from build123d import *

# Parameters (mm, degrees)
BOSS_EXTRUDE1_DEPTH      = 48
CUT_EXTRUDE4_DEPTH       = 2
CUT_EXTRUDE6_DEPTH       = 9
CUT_EXTRUDE6_DEPTH_BACK  = 1
SKETCH8_RX               = 1.5
SKETCH8_RY               = 0.8
CUT_EXTRUDE7_DEPTH       = 11
CUT_EXTRUDE7_DEPTH_BACK  = 1
SKETCH13_RX              = 1.5
SKETCH13_RY              = 0.8
CUT_EXTRUDE8_DEPTH       = 13
CUT_EXTRUDE8_DEPTH_BACK  = 1
SKETCH14_RX              = 1.5
SKETCH14_RY              = 0.8
CUT_EXTRUDE9_DEPTH       = 15
CUT_EXTRUDE9_DEPTH_BACK  = 1
SKETCH15_RX              = 1.5
SKETCH15_RY              = 0.8
CUT_EXTRUDE10_DEPTH      = 17
CUT_EXTRUDE10_DEPTH_BACK = 1
SKETCH16_RX              = 1.5
SKETCH16_RY              = 0.8
CUT_EXTRUDE11_DEPTH      = 19
CUT_EXTRUDE11_DEPTH_BACK = 1
SKETCH17_RX              = 1.5
SKETCH17_RY              = 0.8
CUT_EXTRUDE12_DEPTH      = 21
CUT_EXTRUDE12_DEPTH_BACK = 1
SKETCH18_RX              = 1.5
SKETCH18_RY              = 0.8
CUT_EXTRUDE13_DEPTH      = 23
CUT_EXTRUDE13_DEPTH_BACK = 1
SKETCH19_RX              = 1.5
SKETCH19_RY              = 0.8
SKETCH21_W               = 58.141640115
SKETCH21_H               = 26.059597095
CUT_EXTRUDE14_DEPTH      = 22
BODY_MOVE_COPY1_ANGLE    = 180


with BuildPart() as part:
    # Sketch2 → Boss-Extrude1 (new body)
    with BuildSketch(Plane.XY):
        Polygon((-7.23, -20.3), (-7.23, -34), (-9.23, -34), (-9.23, -2), (-7.23, -2), align=None)
    extrude(amount=BOSS_EXTRUDE1_DEPTH)

    # Sketch7 → Cut-Extrude4 (cut)
    with BuildSketch(Plane(origin=(-7.23, 0, 0), x_dir=(0, 0, -1), z_dir=(1, 0, 0))):
        Polygon((-48, -16.3), (-48, -24.3), (-42, -24.3), (-42, -25.3), (-36, -25.3), (-36, -26.3), (-30, -26.3), (-30, -27.3), (-24, -27.3), (-24, -28.3), (-18, -28.3), (-18, -29.3), (-12, -29.3), (-12, -30.3), (-6, -30.3), (-6, -31.3), (0, -31.3), (0, -9.3), (-6, -9.3), (-6, -10.3), (-12, -10.3), (-12, -11.3), (-18, -11.3), (-18, -12.3), (-24, -12.3), (-24, -13.3), (-30, -13.3), (-30, -14.3), (-36, -14.3), (-36, -15.3), (-42, -15.3), (-42, -16.3), align=None)
    extrude(amount=-CUT_EXTRUDE4_DEPTH, mode=Mode.SUBTRACT)


with BuildPart() as cut_extrude4_piece_1:
    # of the separate pieces the step leaves, piece 1, a body of its own (cut_extrude4_pieces)
    add(part.part.solids().sort_by_distance((-7.23, -9.3, 0))[0])


with BuildPart() as cut_extrude4_piece_2:
    # of the separate pieces the step leaves, piece 2, a body of its own (cut_extrude4_pieces)
    add(part.part.solids().sort_by_distance((-7.23, -34, 0))[0])


with BuildPart() as cut_extrude6_tool:
    # Sketch8 → Cut-Extrude6 (new, two sides: drawn at the far end of the back side and taken through both)
    with BuildSketch(Plane(origin=(0, -24.3, 0), x_dir=(1, 0, 0), z_dir=(0, 1, 0)).offset(-CUT_EXTRUDE6_DEPTH_BACK)):
        with Locations(Location((-8.23, -45), (0, 0, 90))):
            Ellipse(SKETCH8_RX, SKETCH8_RY)
    extrude(amount=CUT_EXTRUDE6_DEPTH + CUT_EXTRUDE6_DEPTH_BACK)


with BuildPart() as cut_extrude4_piece_1_1:
    add(cut_extrude4_piece_1.part)

    # Cut-Extrude6: cut by cut_extrude6_tool
    add(cut_extrude6_tool.part, mode=Mode.SUBTRACT)


with BuildPart() as cut_extrude4_piece_2_1:
    add(cut_extrude4_piece_2.part)

    # Cut-Extrude6: cut by cut_extrude6_tool
    add(cut_extrude6_tool.part, mode=Mode.SUBTRACT)


with BuildPart() as cut_extrude7_tool:
    # Sketch13 → Cut-Extrude7 (new, two sides: drawn at the far end of the back side and taken through both)
    with BuildSketch(Plane(origin=(0, -25.3, 0), x_dir=(1, 0, 0), z_dir=(0, 1, 0)).offset(-CUT_EXTRUDE7_DEPTH_BACK)):
        with Locations(Location((-8.23, -39), (0, 0, 90))):
            Ellipse(SKETCH13_RX, SKETCH13_RY)
    extrude(amount=CUT_EXTRUDE7_DEPTH + CUT_EXTRUDE7_DEPTH_BACK)


with BuildPart() as cut_extrude4_piece_1_2:
    add(cut_extrude4_piece_1_1.part)

    # Cut-Extrude7: cut by cut_extrude7_tool
    add(cut_extrude7_tool.part, mode=Mode.SUBTRACT)


with BuildPart() as cut_extrude4_piece_2_2:
    add(cut_extrude4_piece_2_1.part)

    # Cut-Extrude7: cut by cut_extrude7_tool
    add(cut_extrude7_tool.part, mode=Mode.SUBTRACT)


with BuildPart() as cut_extrude8_tool:
    # Sketch14 → Cut-Extrude8 (new, two sides: drawn at the far end of the back side and taken through both)
    with BuildSketch(Plane(origin=(0, -26.3, 0), x_dir=(1, 0, 0), z_dir=(0, 1, 0)).offset(-CUT_EXTRUDE8_DEPTH_BACK)):
        with Locations(Location((-8.23, -33), (0, 0, 90))):
            Ellipse(SKETCH14_RX, SKETCH14_RY)
    extrude(amount=CUT_EXTRUDE8_DEPTH + CUT_EXTRUDE8_DEPTH_BACK)


with BuildPart() as cut_extrude4_piece_1_3:
    add(cut_extrude4_piece_1_2.part)

    # Cut-Extrude8: cut by cut_extrude8_tool
    add(cut_extrude8_tool.part, mode=Mode.SUBTRACT)


with BuildPart() as cut_extrude4_piece_2_3:
    add(cut_extrude4_piece_2_2.part)

    # Cut-Extrude8: cut by cut_extrude8_tool
    add(cut_extrude8_tool.part, mode=Mode.SUBTRACT)


with BuildPart() as cut_extrude9_tool:
    # Sketch15 → Cut-Extrude9 (new, two sides: drawn at the far end of the back side and taken through both)
    with BuildSketch(Plane(origin=(0, -27.3, 0), x_dir=(1, 0, 0), z_dir=(0, 1, 0)).offset(-CUT_EXTRUDE9_DEPTH_BACK)):
        with Locations(Location((-8.23, -27), (0, 0, 90))):
            Ellipse(SKETCH15_RX, SKETCH15_RY)
    extrude(amount=CUT_EXTRUDE9_DEPTH + CUT_EXTRUDE9_DEPTH_BACK)


with BuildPart() as cut_extrude4_piece_1_4:
    add(cut_extrude4_piece_1_3.part)

    # Cut-Extrude9: cut by cut_extrude9_tool
    add(cut_extrude9_tool.part, mode=Mode.SUBTRACT)


with BuildPart() as cut_extrude4_piece_2_4:
    add(cut_extrude4_piece_2_3.part)

    # Cut-Extrude9: cut by cut_extrude9_tool
    add(cut_extrude9_tool.part, mode=Mode.SUBTRACT)


with BuildPart() as cut_extrude10_tool:
    # Sketch16 → Cut-Extrude10 (new, two sides: drawn at the far end of the back side and taken through both)
    with BuildSketch(Plane(origin=(0, -28.3, 0), x_dir=(1, 0, 0), z_dir=(0, 1, 0)).offset(-CUT_EXTRUDE10_DEPTH_BACK)):
        with Locations(Location((-8.23, -21), (0, 0, 90))):
            Ellipse(SKETCH16_RX, SKETCH16_RY)
    extrude(amount=CUT_EXTRUDE10_DEPTH + CUT_EXTRUDE10_DEPTH_BACK)


with BuildPart() as cut_extrude4_piece_1_5:
    add(cut_extrude4_piece_1_4.part)

    # Cut-Extrude10: cut by cut_extrude10_tool
    add(cut_extrude10_tool.part, mode=Mode.SUBTRACT)


with BuildPart() as cut_extrude4_piece_2_5:
    add(cut_extrude4_piece_2_4.part)

    # Cut-Extrude10: cut by cut_extrude10_tool
    add(cut_extrude10_tool.part, mode=Mode.SUBTRACT)


with BuildPart() as cut_extrude11_tool:
    # Sketch17 → Cut-Extrude11 (new, two sides: drawn at the far end of the back side and taken through both)
    with BuildSketch(Plane(origin=(0, -29.3, 0), x_dir=(1, 0, 0), z_dir=(0, 1, 0)).offset(-CUT_EXTRUDE11_DEPTH_BACK)):
        with Locations(Location((-8.23, -15), (0, 0, 90))):
            Ellipse(SKETCH17_RX, SKETCH17_RY)
    extrude(amount=CUT_EXTRUDE11_DEPTH + CUT_EXTRUDE11_DEPTH_BACK)


with BuildPart() as cut_extrude4_piece_1_6:
    add(cut_extrude4_piece_1_5.part)

    # Cut-Extrude11: cut by cut_extrude11_tool
    add(cut_extrude11_tool.part, mode=Mode.SUBTRACT)


with BuildPart() as cut_extrude4_piece_2_6:
    add(cut_extrude4_piece_2_5.part)

    # Cut-Extrude11: cut by cut_extrude11_tool
    add(cut_extrude11_tool.part, mode=Mode.SUBTRACT)


with BuildPart() as cut_extrude12_tool:
    # Sketch18 → Cut-Extrude12 (new, two sides: drawn at the far end of the back side and taken through both)
    with BuildSketch(Plane(origin=(0, -30.3, 0), x_dir=(1, 0, 0), z_dir=(0, 1, 0)).offset(-CUT_EXTRUDE12_DEPTH_BACK)):
        with Locations(Location((-8.23, -9), (0, 0, 90))):
            Ellipse(SKETCH18_RX, SKETCH18_RY)
    extrude(amount=CUT_EXTRUDE12_DEPTH + CUT_EXTRUDE12_DEPTH_BACK)


with BuildPart() as cut_extrude4_piece_1_7:
    add(cut_extrude4_piece_1_6.part)

    # Cut-Extrude12: cut by cut_extrude12_tool
    add(cut_extrude12_tool.part, mode=Mode.SUBTRACT)


with BuildPart() as cut_extrude4_piece_2_7:
    add(cut_extrude4_piece_2_6.part)

    # Cut-Extrude12: cut by cut_extrude12_tool
    add(cut_extrude12_tool.part, mode=Mode.SUBTRACT)


with BuildPart() as cut_extrude13_tool:
    # Sketch19 → Cut-Extrude13 (new, two sides: drawn at the far end of the back side and taken through both)
    with BuildSketch(Plane(origin=(0, -31.3, 0), x_dir=(1, 0, 0), z_dir=(0, 1, 0)).offset(-CUT_EXTRUDE13_DEPTH_BACK)):
        with Locations(Location((-8.23, -3), (0, 0, 90))):
            Ellipse(SKETCH19_RX, SKETCH19_RY)
    extrude(amount=CUT_EXTRUDE13_DEPTH + CUT_EXTRUDE13_DEPTH_BACK)


with BuildPart() as cut_extrude4_piece_1_8:
    add(cut_extrude4_piece_1_7.part)

    # Cut-Extrude13: cut by cut_extrude13_tool
    add(cut_extrude13_tool.part, mode=Mode.SUBTRACT)


with BuildPart() as cut_extrude4_piece_2_8:
    add(cut_extrude4_piece_2_7.part)

    # Cut-Extrude13: cut by cut_extrude13_tool
    add(cut_extrude13_tool.part, mode=Mode.SUBTRACT)

    # Sketch21 → Cut-Extrude14 (cut)
    with BuildSketch(Plane(origin=(0, 0, 0), x_dir=(0, 0, -1), z_dir=(1, 0, 0))):
        with Locations((-20.055207527, -35.194061722)):
            Rectangle(SKETCH21_W, SKETCH21_H)
    extrude(amount=-CUT_EXTRUDE14_DEPTH, mode=Mode.SUBTRACT)


with BuildPart() as cut_extrude4_piece_1_9:
    # Body-Move/Copy1: moved
    add(cut_extrude4_piece_1_8.part.rotate(Axis((-8.23, -9.15, 0), (0, 0, 1)), BODY_MOVE_COPY1_ANGLE))


solid = cut_extrude4_piece_1_9.part
Work out the finished part from the listing and answer in its coordinate system (mm). A direction names the side the tool comes from. Give positions to 0.01 mm unless a question says otherwise; leave off trailing zeros. Write each loop counter-clockwise with the first axis right and the second up, starting at its lowest first coordinate (ties: lowest second). Pieces come first, ordered by that corner, then holes. Notation, with made-up numbers: (40, -34.5) - (79, -34.5) arc R24 cw to (79, -8.5) - close; hole circle Ø5 at (-11.75, -37.5). An arc over 180 degrees is marked (long way). One line per item, written item: value. Start each with the question number.
1. For a pull along X with two mould halves and no side action, classify faces 1 (the flat face through (-9, -6, 20)), 2 (the flat face through (-8, -4, 39)), 3 (the flat face through (-7.23, -11, 24)) as +X half, -X half, draft (parallel to the pull), parting line (faces both ways), or undercut.
2. Find section B-B (z = 29). Write down the section's boundary in (x, y).
3. Consider probe 1 along Y at (x, z) = (-8.6, 7.5); probe 2 along Y at (x, z) = (-8.85, 5); probe 3 along Z at (x, y) = (-8.05, -9.75). Determine where each line is inside the solid, lowest interval first.
4. For faces 4 (the flat face through (-8, -5, 33)), 5 (the flat face through (-8.2, -4.5, 30)), 6 (the flat face through (-8, -16.3, 24)), determine the directions among +Z, -Z, +X, -X, +Y, -Y from which every point of the face is accessible in a straight line to the end or side of a thin tool.
5. Find section A-A (z = 7). Write down the section's boundary in (x, y).
6. Given pin 1 (0.8 mm diameter, centred on x = -8, z = 33.5, fed in from +Y); pin 2 (0.5 mm diameter, centred on x = -8, y = -2.5, fed in from -Z); pin 3 (1.1 mm diameter, centred on x = -8.5, y = -5.5, fed in from -Z), each flat-ended and moving along its own axis, determine where each tip first touches the part or whether it passes through.
Geometry results:
1. face 1: draft
1. face 2: undercut
1. face 3: +X half
2. outline: (-9.23, -16.3) - (-7.23, -16.3) - (-7.23, -5) - (-9.23, -5) - close
3. probe 1: -16.3 to -8
3. probe 2: -16.3 to -9
3. probe 3: 0 to 1.54, 4.46 to 48
4. face 4: +Y
4. face 5: -Z, +X, -X, +Y
4. face 6: +Z, -Z, +X, -X, -Y
5. outline: (-9.23, -16.3) - (-7.23, -16.3) - (-7.23, -8) - (-9.23, -8) - close
6. pin 1: y = -5
6. pin 2: z = 42
6. pin 3: z = 18
